Geometry: see drawing. Coordinates: mm, zero at the bounding-box minimum. A direction names the side the tool comes from. Round coordinates to 2 decimals unless told otherwise and drop trailing zeros. Write each loop counter-clockwise with the first axis right and the second up, starting at its lowest first coordinate (ties: lowest second). Pieces come first, ordered by that corner, then holes. Notation, with made-up numbers: (0.5, 24.5) -> (58.5, 24.5) arc R9 ccw to (58.5, 41.5) -> close; hole circle Ø2 at (41.5, 47). An arc over 180 degrees is marked (long way). Write item = value, one per line.
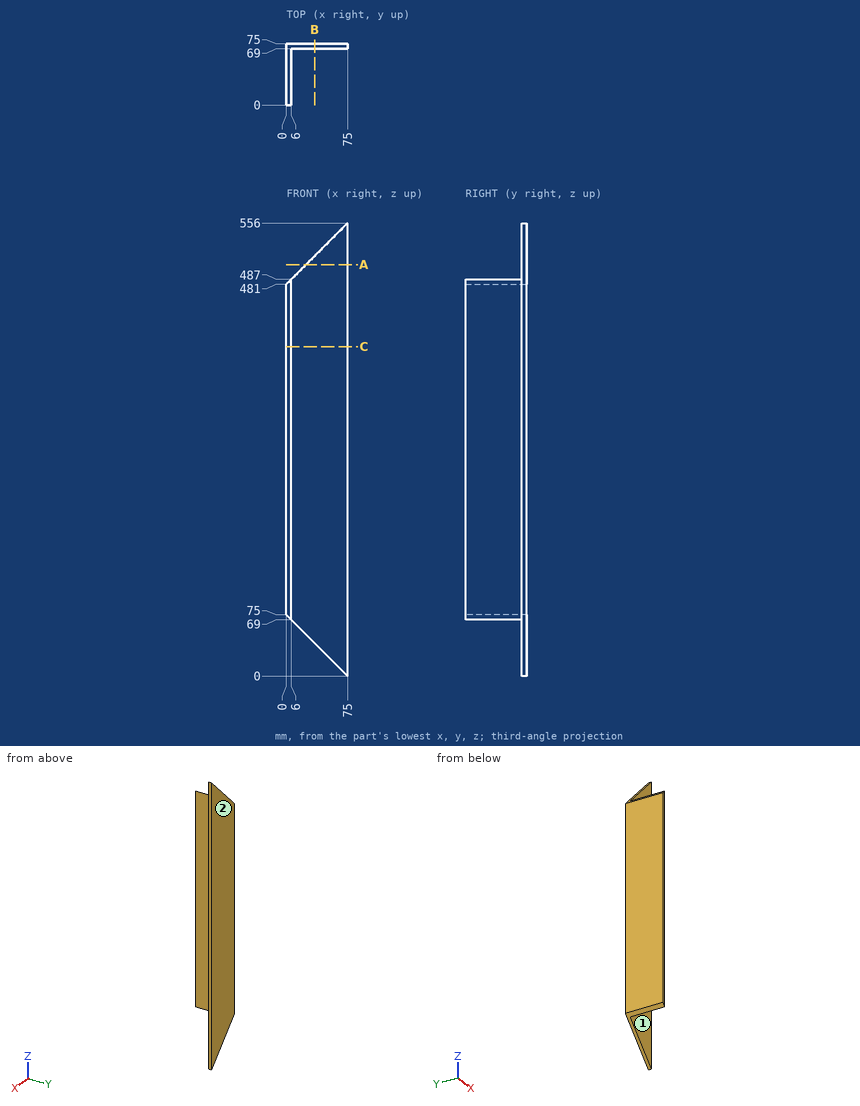
1) Cut plane A-A (z = 505). Return the cut outline in (x, y), and give its area (3 significant figures).
Solutions:
outline = (24, 69) -> (75, 69) -> (75, 75) -> (24, 75) -> close
area = 306 mm^2
2) Cut plane B-B (x = 34.5). Return the cut outline in (y, z).
Solutions:
outline = (69, 40.5) -> (75, 40.5) -> (75, 515.5) -> (69, 515.5) -> close
3) Line query: L1, parallel to X at y = 19, z = 81; L2, parallel to Y at x = 29, z = 237.5; L3, parallel to Z at x = 23.5, y = 71. Output: solid intervals per line, ascending. Write a range as from..to.
Solutions:
L1 = 0..6
L2 = 69..75
L3 = 51.5..504.5
4) Cut plane C-C (z = 404.5). Return the cut outline in (x, y).
Solutions:
outline = (0, 0) -> (6, 0) -> (6, 69) -> (75, 69) -> (75, 75) -> (0, 75) -> close
5) Access query for the marked faces 1 and 2. Directions: +Z, -Z, +X, -X, +Y, -Y. A direction counts if a zero-diameter tool reaches every point of the face in a straight line with its end or side. Return the directions, or none.
Solutions:
face_1 = +Z, -Z, +X, -Y
face_2 = +Z, -Z, +X, -X, +Y
6) First-contact query: P1, Ø20.5, axis at y = 45, z = 198, coming from the +X side; P2, Ø4, axis at x = 37.5, z = 459, coming from the -Y side. Flat tips, straight axial feed; report the tip coordinate or a pass-through.
Solutions:
P1 = 6
P2 = 69
